```python
from build123d import *

# Parameters (mm, degrees)
SKETCH1_W           = 42.3
SKETCH1_H           = 42.3
SKETCH1_R           = 1.6
BOSS_EXTRUDE1_DEPTH = 40
SKETCH2_R           = 15
CUT_EXTRUDE1_DEPTH  = 40
CHAMFER1_SIZE       = 4
CHAMFER2_SIZE       = 2
SKETCH3_W           = 30
SKETCH3_H           = 20
CUT_EXTRUDE2_DEPTH  = 72.962351268
SKETCH4_W           = 20
SKETCH4_H           = 30
CUT_EXTRUDE3_DEPTH  = 72.962351268
CHAMFER3_SIZE       = 2
SKETCH5_W           = 30
SKETCH5_H           = 15
CUT_EXTRUDE5_DEPTH  = 2
CIRPATTERN1_COUNT   = 4
CUT_EXTRUDE6_DEPTH  = 2
CIRPATTERN2_COUNT   = 4
CUT_EXTRUDE7_DEPTH  = 20
CIRPATTERN3_COUNT   = 4
SKETCH10_R          = 3
CUT_EXTRUDE8_DEPTH  = 20


with BuildPart() as part:
    # Sketch1 → Boss-Extrude1 (new body)
    with BuildSketch(Plane.XY):
        with Locations((21.15, 21.15)):
            Rectangle(SKETCH1_W, SKETCH1_H)
        with Locations((5.65, 36.65)):
            Circle(SKETCH1_R, mode=Mode.SUBTRACT)
        with Locations((5.65, 5.65)):
            Circle(SKETCH1_R, mode=Mode.SUBTRACT)
        with Locations((36.65, 5.65)):
            Circle(SKETCH1_R, mode=Mode.SUBTRACT)
        with Locations((36.65, 36.65)):
            Circle(SKETCH1_R, mode=Mode.SUBTRACT)
    extrude(amount=BOSS_EXTRUDE1_DEPTH)

    # Sketch2 → Cut-Extrude1 (cut)
    with BuildSketch(Plane.XY.offset(40)):
        with Locations((21.15, 21.15)):
            Circle(SKETCH2_R)
    extrude(amount=-CUT_EXTRUDE1_DEPTH, mode=Mode.SUBTRACT)

    # Chamfer1
    chamfer1_edges = [part.edges().sort_by_distance(p)[0] for p in [
        (0, 0, 20),
        (0, 42.3, 20),
        (42.3, 42.3, 20),
        (42.3, 0, 20),
    ]]
    chamfer(chamfer1_edges, length=CHAMFER1_SIZE)

    # Chamfer2
    chamfer2_edges = [part.edges().sort_by_distance(p)[0] for p in [
        (6.15, 21.15, 0),
        (6.15, 21.15, 40),
    ]]
    chamfer(chamfer2_edges, length=CHAMFER2_SIZE)

    # Sketch3 → Cut-Extrude2 (cut, through all)
    with BuildSketch(Plane(origin=(42.3, 0, 0), x_dir=(0, 0, -1), z_dir=(1, 0, 0))):
        with Locations((-20, 21.15)):
            Rectangle(SKETCH3_W, SKETCH3_H)
    extrude(amount=-CUT_EXTRUDE2_DEPTH, mode=Mode.SUBTRACT)

    # Sketch4 → Cut-Extrude3 (cut, through all)
    with BuildSketch(Plane(origin=(0, 42.3, 0), x_dir=(1, 0, 0), z_dir=(0, 1, 0))):
        with Locations((21.15, -20)):
            Rectangle(SKETCH4_W, SKETCH4_H)
    extrude(amount=-CUT_EXTRUDE3_DEPTH, mode=Mode.SUBTRACT)

    # Chamfer3
    chamfer3_edges = [part.edges().sort_by_distance(p)[0] for p in [
        (31.15, 37.315169944, 5),
        (31.15, 4.984830056, 5),
        (31.15, 4.984830056, 35),
        (31.15, 37.315169944, 35),
        (11.15, 4.984830056, 35),
        (11.15, 37.315169944, 35),
        (11.15, 4.984830056, 5),
        (11.15, 37.315169944, 5),
        (4.984830056, 31.15, 5),
        (37.315169944, 31.15, 5),
        (37.315169944, 11.15, 5),
        (4.984830056, 11.15, 5),
        (4.984830056, 11.15, 35),
        (37.315169944, 11.15, 35),
        (4.984830056, 31.15, 35),
        (37.315169944, 31.15, 35),
    ]]
    chamfer(chamfer3_edges, length=CHAMFER3_SIZE)

    # Sketch5 → Cut-Extrude5 (cut)
    with BuildSketch(Plane(origin=(-19.15, 19.15, 0), x_dir=(0, 0, 1), z_dir=(-0.7071067811865469, 0.7071067811865481, 0))):
        with Locations((20, 29.910616844)):
            Rectangle(SKETCH5_W, SKETCH5_H)
    cut_extrude5 = extrude(amount=-CUT_EXTRUDE5_DEPTH, mode=Mode.SUBTRACT)

    # CirPattern1: Cut-Extrude5 ×4 about axis
    cirpattern1_axis = Axis((21.15, 21.15, 0), (0, 0, 1))
    for i in range(1, CIRPATTERN1_COUNT):
        add(cut_extrude5.rotate(cirpattern1_axis, i * 360 / CIRPATTERN1_COUNT), mode=Mode.SUBTRACT)

    # Sketch8 → Cut-Extrude6 (cut)
    with BuildSketch(Plane.XY.offset(5)):
        Polygon((36.821572875, 40.95), (32.35, 40.95), (32.35, 32.35), (40.95, 32.35), (40.95, 36.821572875), align=None)
        Polygon((35.471572875, 42.3), (36.821572875, 40.95), (39.65, 40.95), (38.3, 42.3), align=None)
        Polygon((32.35, 42.3), (32.35, 40.95), (36.821572875, 40.95), (35.471572875, 42.3), align=None)
        Polygon((39.65, 40.95), (36.821572875, 40.95), (40.95, 36.821572875), (40.95, 39.65), align=None)
        Polygon((38.3, 42.3), (39.65, 40.95), (40.95, 40.95), (40.95, 42.3), align=None)
    cut_extrude6 = extrude(amount=CUT_EXTRUDE6_DEPTH, mode=Mode.SUBTRACT)

    # CirPattern2: Cut-Extrude6 ×4 about axis
    cirpattern2_axis = Axis((21.15, 21.15, 0), (0, 0, 1))
    for i in range(1, CIRPATTERN2_COUNT):
        add(cut_extrude6.rotate(cirpattern2_axis, i * 360 / CIRPATTERN2_COUNT), mode=Mode.SUBTRACT)

    # Sketch9 → Cut-Extrude7 (cut)
    with BuildSketch(Plane(origin=(0, 0, 35), x_dir=(-1, 0, 0), z_dir=(0, 0, -1))):
        with BuildLine():
            Line((-36.65, 32.9), (-42.3, 32.9))
            Line((-42.3, 32.9), (-42.3, 38.3))
            Line((-42.3, 38.3), (-38.3, 42.3))
            Line((-38.3, 42.3), (-32.9, 42.3))
            Line((-32.9, 42.3), (-32.9, 36.65))
            ThreePointArc((-32.9, 36.65), (-33.998349571, 33.998349571), (-36.65, 32.9))
        make_face()
    cut_extrude7 = extrude(amount=CUT_EXTRUDE7_DEPTH, mode=Mode.SUBTRACT)

    # CirPattern3: Cut-Extrude7 ×4 about axis
    cirpattern3_axis = Axis((21.15, 21.15, 0), (0, 0, 1))
    for i in range(1, CIRPATTERN3_COUNT):
        add(cut_extrude7.rotate(cirpattern3_axis, i * 360 / CIRPATTERN3_COUNT), mode=Mode.SUBTRACT)

    # Sketch10 → Cut-Extrude8 (cut)
    with BuildSketch(Plane(origin=(0, 0, 0), x_dir=(-1, 0, 0), z_dir=(0, 0, -1))):
        with Locations((-36.65, 36.65)):
            Circle(SKETCH10_R)
        with Locations((-5.65, 36.65)):
            Circle(SKETCH10_R)
        with Locations((-5.65, 5.65)):
            Circle(SKETCH10_R)
        with Locations((-36.65, 5.65)):
            Circle(SKETCH10_R)
    extrude(amount=-CUT_EXTRUDE8_DEPTH, mode=Mode.SUBTRACT)


solid = part.part
```
Here's how the part is built. I have some questions about the finished solid (model axes, mm). A direction names the side the tool comes from. Round coordinates to 2 decimals unless told otherwise and drop trailing zeros. Write each loop counter-clockwise with the first axis right and the second up, starting at its lowest first coordinate (ties: lowest second). Pieces come first, ordered by that corner, then holes. Notation, with made-up numbers: M -23.5,80 L 4.5,80 A20 ccw 4.5,119 Z; hole C -16,43.25 d8. An arc over 180 degrees is marked long. Answer as CSV lines item,"result". Start each with the question number.
1. On a 3-axis mill with a long thin cutter (end or side, diameter ignored), from which of +Z, -Z, +X, -X, +Y, -Y can I reach the whole of each face in a straight line? I mean faces 4 (the flat face through (9.4, 39, 25)), 5 (the flat face through (21, 3, 5)), 6 (the flat face through (39.4, 3.7, 5)). Say none if no direction works.
2. Thinking about a two-plate mould opening in Y: for faces 1 (the flat face through (39, 32.9, 25)), 2 (the flat face through (12.14, 37.38, 33.99)), 3 (the flat face through (5.05, 30.14, 5.99)), which applies, released by +Y, released by -Y, zero draft, split by the parting line, or undercut?
3. Suppose I cut it at A-A on z = 12. Write out the boundary of the cut face in (x, y).
4. I'm going to push flat-ended pins straight in: pin 1 Ø1.9 at (x, y) = (5.65, 5.65) entering from +Z; pin 2 Ø0.6 at (x, z) = (4.5, 6) entering from +Y; pin 3 Ø1 at (y, z) = (38, 6) entering from +X; pin 4 Ø4.5 at (x, z) = (38.5, 27.5) entering from -Y. Where does each tip first touch, or does it pass through?
5. Suppose I cut it at B-B on x = 21.15. Write out the boundary of the cut face in (y, z).
6. Suppose I cut it at C-C on z = 34. Count the separate pieces of the cut face and the enclosed holes in it, then the cut area to 3 significant figures.
7. I need wall thicknesses on probe 1 along Z at (x, y) = (5, 40); probe 2 along Y at (x, z) = (36.65, 36.5); probe 3 along Y at (x, z) = (39, 20). Which ranges of each line are inside material? Lowest first, please.
8. Suppose I cut it at D-D on z = 3. Write out the boundary of the cut face in (x, y).
Check result:
1,face 4,"-X, +Y"
1,face 5,"+Y, -Y"
1,face 6,"+X"
2,face 1,"released by +Y"
2,face 2,"zero draft"
2,face 3,"undercut"
3,outline,"M 0,6.83 L 6.83,0 L 11.15,0 L 11.15,9.97 A15 cw 9.97,11.15 L 0,11.15 Z; M 0,31.15 L 9.97,31.15 A15 cw 11.15,32.33 L 11.15,42.3 L 6.83,42.3 L 0,35.47 Z; M 31.15,0 L 35.47,0 L 42.3,6.83 L 42.3,11.15 L 32.33,11.15 A15 cw 31.15,9.97 Z; M 31.15,32.33 A15 cw 32.33,31.15 L 42.3,31.15 L 42.3,35.47 L 35.47,42.3 L 31.15,42.3 Z; hole C 5.65,5.65 d6; hole C 5.65,36.65 d6; hole C 36.65,5.65 d6; hole C 36.65,36.65 d6"
4,pin 1,"passes through"
4,pin 2,"stops at y = 32.35"
4,pin 3,"stops at x = 32.35"
4,pin 4,"stops at y = 9.38"
5,outline,"M 0,0 L 4.15,0 L 6.15,2 L 6.15,5 L 0,5 Z; M 0,35 L 6.15,35 L 6.15,38 L 4.15,40 L 0,40 Z; M 36.15,2 L 38.15,0 L 42.3,0 L 42.3,5 L 36.15,5 Z; M 36.15,35 L 42.3,35 L 42.3,40 L 38.15,40 L 36.15,38 Z"
6,separate pieces,"4"
6,enclosed holes,"0"
6,area,"229 mm2"
7,probe 1,"z = 0 to 5, 7 to 15, 35 to 40"
7,probe 2,"y = 0 to 4.05, 7.25 to 35.05, 38.25 to 42.3"
7,probe 3,"y = 9.4 to 11.15, 31.15 to 32.9"
8,outline,"M 0,4 L 4,0 L 38.3,0 L 42.3,4 L 42.3,38.3 L 38.3,42.3 L 4,42.3 L 0,38.3 Z; hole C 5.65,5.65 d6; hole C 5.65,36.65 d6; hole C 21.15,21.15 d30; hole C 36.65,5.65 d6; hole C 36.65,36.65 d6"
